```python
from build123d import *

# Parameters (mm, degrees)
SKETCH_1_W          = 50
SKETCH_1_H          = 35
EXTRUDE_1_DEPTH     = 2.2
SKETCH_2_R          = 8
CUT_EXTRUDE_1_DEPTH = 2.2
SKETCH_3_W          = 50
SKETCH_3_H          = 2.2
EXTRUDE_2_DEPTH     = 13.8
SKETCH_4_R          = 1.65
CUT_EXTRUDE_2_DEPTH = 13.8


with BuildPart() as part:
    # 草图1 → 凸台-拉伸1 (new body)
    with BuildSketch(Plane.XY):
        with Locations((25, 17.5)):
            Rectangle(SKETCH_1_W, SKETCH_1_H)
    extrude(amount=EXTRUDE_1_DEPTH)

    # 草图2 → 切除-拉伸1 (cut)
    with BuildSketch(Plane.XY.offset(2.2)):
        with Locations((12, 22.5)):
            Circle(SKETCH_2_R)
        with Locations((38, 22.5)):
            Circle(SKETCH_2_R)
    extrude(amount=-CUT_EXTRUDE_1_DEPTH, mode=Mode.SUBTRACT)

    # 草图3 → 凸台-拉伸2 (add)
    with BuildSketch(Plane.XY.offset(2.2)):
        with Locations((25, 1.1)):
            Rectangle(SKETCH_3_W, SKETCH_3_H)
    extrude(amount=EXTRUDE_2_DEPTH)

    # 草图4 → 切除-拉伸2 (cut)
    with BuildSketch(Plane(origin=(0, 2.2, 0), x_dir=(1, 0, 0), z_dir=(0, 1, 0))):
        with Locations(Location((18.15, -9.1, 0), (0, 0, 270))):
            Circle(SKETCH_4_R)
        with Locations(Location((31.85, -9.1, 0), (0, 0, 270))):
            Circle(SKETCH_4_R)
    extrude(amount=-CUT_EXTRUDE_2_DEPTH, mode=Mode.SUBTRACT)


solid = part.part
```
Source: CAD feature listing. Evaluate the final solid. Frame: model axes, mm. A direction names the side the tool comes from. Give positions to 0.01 mm unless a question says otherwise; leave off trailing zeros. Loops run counter-clockwise (first coordinate to the right, second up) from the corner with the lowest first, then second, coordinate; pieces in that order, holes last. Notation, with made-up numbers: (57.5, 62.5) -> (66.5, 62.5) arc R10 cw to (66.5, 79.5) -> close; hole circle Ø8 at (63, -15). An arc over 180 degrees is marked (long way). Use a Markdown table: item, result. Add a question column.
(1) Section query A-A (y = 22.5). Output: boundary loops of the cut face in (x, z).
(2) Ray query, line 1 (X direction, y = 1.65, z = 9.1); line 2 (Z direction, x = 18, y = 1); line 3 (Y direction, x = 12, z = 1.25). Return the intervals inside material, ascending.
(3) First-contact query: pin 1 Ø1.5 at (y, z) = (23, 3.5) entering from -X; pin 2 Ø7 at (x, z) = (15.5, 11) entering from +Y; pin 3 Ø10 at (x, y) = (7, 14) entering from +Z. Flat tips, straight axial feed; report the tip coordinate or a pass-through.
(4) Section query C-C (x = 38). Output: boundary loops of the cut face in (y, z), then the cut area to 3 significant figures.
(5) Pull-direction query (Y, two-part tool) for faces 3 (the face through (10.959, 30.432, 1.115)), 4 (the face through (25, 2.2, 9)), 5 (the face through (0, 12, 2)), 6 (the face through (32.1, 27.9, 1.1)); classes: +Y half, -Y half, draft (parallel to the pull), parting line (faces both ways), or undercut.
(6) Section query B-B (z = 9.1). Output: boundary loops of the cut face in (x, y).
(7) Section query D-D (x = 31.85). Output: boundary loops of the cut face in (y, z).
(8) Access query for faces 1 (the face through (25, 19, 2.2)), 2 (the face through (25, 18, 0)). Directions: +Z, -Z, +X, -X, +Y, -Y. A direction counts if a zero-diameter tool reaches every point of the face in a straight line with its end or side. Return the directions, or none.
Checked values:
| question | item | result |
|---|---|---|
| 1 | outline | (0, 0) -> (4, 0) -> (4, 2.2) -> (0, 2.2) -> close; (20, 0) -> (30, 0) -> (30, 2.2) -> (20, 2.2) -> close; (46, 0) -> (50, 0) -> (50, 2.2) -> (46, 2.2) -> close |
| 2 | line 1 | 0 to 16.5, 19.8 to 30.2, 33.5 to 50 |
| 2 | line 2 | 0 to 7.46, 10.74 to 16 |
| 2 | line 3 | 0 to 14.5, 30.5 to 35 |
| 3 | pin 1 | through |
| 3 | pin 2 | y = 2.2 |
| 3 | pin 3 | z = 2.2 |
| 4 | outline | (0, 0) -> (14.5, 0) -> (14.5, 2.2) -> (2.2, 2.2) -> (2.2, 16) -> (0, 16) -> close; (30.5, 0) -> (35, 0) -> (35, 2.2) -> (30.5, 2.2) -> close |
| 4 | area | 72.2 mm^2 |
| 5 | face 3 | undercut |
| 5 | face 4 | +Y half |
| 5 | face 5 | draft |
| 5 | face 6 | undercut |
| 6 | outline | (0, 0) -> (16.5, 0) -> (16.5, 2.2) -> (0, 2.2) -> close; (19.8, 0) -> (30.2, 0) -> (30.2, 2.2) -> (19.8, 2.2) -> close; (33.5, 0) -> (50, 0) -> (50, 2.2) -> (33.5, 2.2) -> close |
| 7 | outline | (0, 0) -> (17.38, 0) -> (17.38, 2.2) -> (2.2, 2.2) -> (2.2, 7.45) -> (0, 7.45) -> close; (0, 10.75) -> (2.2, 10.75) -> (2.2, 16) -> (0, 16) -> close; (27.62, 0) -> (35, 0) -> (35, 2.2) -> (27.62, 2.2) -> close |
| 8 | face 1 | +Z, +X, -X, +Y |
| 8 | face 2 | -Z, +X, -X, +Y, -Y |
